Could you check a few things on this model? Use its own coordinates, in mm. Face numbers are marked on the shaded views. A direction names the side the tool comes from. Coordinates: 2 decimals unless noted, no trailing zeros. Loops run counter-clockwise (first coordinate to the right, second up) from the corner with the lowest first, then second, coordinate; pieces in that order, holes last.
1) For the marked faces 4, 5 and 6, which set-ups out of +Z, -Z, +X, -X, +Y, -Y let a thin tool reach every point of the face, with its end or its side?
2) Imagine slicing it at A-A on x = 6.25. Please give me the cut outline in (y, z), plus the area to 3 significant figures.
3) Thinking about a two-plate mould opening in Z: for the marked faces 1, 2 and 3, which applies, released by +Z, released by -Z, zero draft, split by the parting line, or undercut?
4) Imagine slicing it at B-B on z = 25. Please give me the cut outline in (x, y), plus the area to 3 significant figures.
5) Imagine slicing it at D-D on z = 10. Please give me the cut outline in (x, y), plus the area to 3 significant figures.
6) Imagine slicing it at C-C on y = 8. Please give me the cut outline in (x, z).
7) Will these pins go through, and if not, where does the flat tip stop? P1, Ø12, axis at y = 12, z = 26, coming from the +X side; P2, Ø2, axis at x = 30.5, y = 5.5, coming from the -Z side; P3, Ø11.5, axis at x = 54.5, z = 19, coming from the +Y side; P4, Ø1.7, axis at x = 20, z = 9.5, coming from the +Y side.
8) If I drill on line 1 along X through (y, z) = (3.7, 5); line 2 along X through (y, z) = (31.75, 10); line 3 along Z through (x, y) = (53, 4), over which ranges is the centre line in solid material (lowest first)?
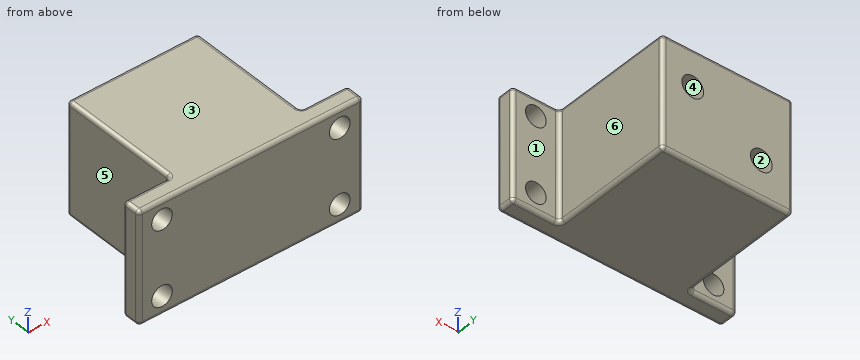
```python
from build123d import *

# Parameters (mm, degrees)
SKETCH2_W           = 60
SKETCH2_H           = 30
BOSS_EXTRUDE1_DEPTH = 5
SKETCH3_W           = 35
SKETCH3_H           = 30
BOSS_EXTRUDE2_DEPTH = 33
SKETCH5_R           = 2.9
CUT_EXTRUDE1_DEPTH  = 20
SKETCH6_R           = 2.75
CUT_EXTRUDE2_DEPTH  = 75.759614766
FILLET1_R           = 1


with BuildPart() as part:
    # Sketch2 → Boss-Extrude1 (new body)
    with BuildSketch(Plane(origin=(0, 0, 0), x_dir=(1, 0, 0), z_dir=(0, 1, 0))):
        with Locations((30, -15)):
            Rectangle(SKETCH2_W, SKETCH2_H)
    extrude(amount=BOSS_EXTRUDE1_DEPTH)

    # Sketch3 → Boss-Extrude2 (add)
    with BuildSketch(Plane(origin=(0, 5, 0), x_dir=(1, 0, 0), z_dir=(0, 1, 0))):
        with Locations((30, -15)):
            Rectangle(SKETCH3_W, SKETCH3_H)
    extrude(amount=BOSS_EXTRUDE2_DEPTH)

    # Sketch5 → Cut-Extrude1 (cut)
    with BuildSketch(Plane(origin=(0, 38, 0), x_dir=(1, 0, 0), z_dir=(0, 1, 0))):
        with Locations(Location((21, -10, 0), (0, 0, 270))):
            Circle(SKETCH5_R)
        with Locations(Location((39.325, -20, 0), (0, 0, 270))):
            Circle(SKETCH5_R)
    extrude(amount=-CUT_EXTRUDE1_DEPTH, mode=Mode.SUBTRACT)

    # Sketch6 → Cut-Extrude2 (cut, through all)
    with BuildSketch(Plane(origin=(0, 5, 0), x_dir=(1, 0, 0), z_dir=(0, 1, 0))):
        with Locations(Location((53.75, -5, 0), (0, 0, 270))):
            Circle(SKETCH6_R)
        with Locations(Location((53.75, -25, 0), (0, 0, 270))):
            Circle(SKETCH6_R)
        with Locations(Location((6.25, -25, 0), (0, 0, 270))):
            Circle(SKETCH6_R)
        with Locations(Location((6.25, -5, 0), (0, 0, 270))):
            Circle(SKETCH6_R)
    extrude(amount=-CUT_EXTRUDE2_DEPTH, mode=Mode.SUBTRACT)

    # Fillet1
    fillet1_edges = [part.edges().sort_by_distance(p)[0] for p in [
        (0, 5, 15),
        (6.25, 5, 0),
        (53.75, 5, 30),
        (6.25, 5, 30),
        (47.5, 5, 15),
        (47.5, 21.5, 30),
        (47.5, 21.5, 0),
        (12.5, 5, 15),
        (12.5, 21.5, 0),
        (12.5, 21.5, 30),
        (47.5, 38, 15),
        (30, 38, 0),
        (12.5, 38, 15),
        (30, 38, 30),
        (60, 5, 15),
        (30, 0, 30),
        (0, 0, 15),
        (30, 0, 0),
        (60, 0, 15),
        (60, 2.5, 30),
        (0, 2.5, 30),
        (0, 2.5, 0),
        (60, 2.5, 0),
        (53.75, 5, 0),
    ]]
    fillet(fillet1_edges, radius=FILLET1_R)


solid = part.part
```
Filled in:
1. face 4: +Y
1. face 5: +Z, -Z, -X, +Y
1. face 6: +Z, -Z, +X, +Y
2. outline: (0, 1) arc R1 ccw to (1, 0) - (4, 0) arc R1 ccw to (5, 1) - (5, 2.25) - (0, 2.25) - close; (0, 7.75) - (5, 7.75) - (5, 22.25) - (0, 22.25) - close; (0, 27.75) - (5, 27.75) - (5, 29) arc R1 ccw to (4, 30) - (1, 30) arc R1 ccw to (0, 29) - close
2. area: 94.1 mm2
3. face 1: zero draft
3. face 2: undercut
3. face 3: released by +Z
4. outline: (0, 1) arc R1 ccw to (1, 0) - (3.5, 0) - (3.5, 5) - (1, 5) arc R1 ccw to (0, 4) - close; (9, 0) - (51, 0) - (51, 5) - (48.5, 5) arc R1 cw to (47.5, 6) - (47.5, 37) arc R1 ccw to (46.5, 38) - (13.5, 38) arc R1 ccw to (12.5, 37) - (12.5, 6) arc R1 cw to (11.5, 5) - (9, 5) - close; (56.5, 0) - (59, 0) arc R1 ccw to (60, 1) - (60, 4) arc R1 ccw to (59, 5) - (56.5, 5) - close
4. area: 1,400 mm2
5. outline: (0, 1) arc R1 ccw to (1, 0) - (59, 0) arc R1 ccw to (60, 1) - (60, 4) arc R1 ccw to (59, 5) - (48.5, 5) arc R1 cw to (47.5, 6) - (47.5, 37) arc R1 ccw to (46.5, 38) - (23.9, 38) - (23.9, 18) - (18.1, 18) - (18.1, 38) - (13.5, 38) arc R1 ccw to (12.5, 37) - (12.5, 6) arc R1 cw to (11.5, 5) - (1, 5) arc R1 ccw to (0, 4) - close
5. area: 1,340 mm2
6. outline: (12.5, 1) arc R1 ccw to (13.5, 0) - (46.5, 0) arc R1 ccw to (47.5, 1) - (47.5, 29) arc R1 ccw to (46.5, 30) - (13.5, 30) arc R1 ccw to (12.5, 29) - close
7. P1: stops at x = 47.5
7. P2: stops at z = 0
7. P3: stops at y = 5
7. P4: stops at y = 18
8. line 1: x = 0 to 3.5, 9 to 51, 56.5 to 60
8. line 2: x = 12.5 to 18.1, 23.9 to 47.5
8. line 3: z = 0 to 2.35, 7.65 to 22.35, 27.65 to 30
